For this review, take the finished solid that the model builds, in its own axes (mm). A direction names the side the tool comes from. Give positions to 0.01 mm unless a question says otherwise; leave off trailing zeros. Write each loop counter-clockwise with the first axis right and the second up, starting at its lowest first coordinate (ties: lowest second). Pieces come first, ordered by that corner, then holes. Notation, with made-up numbers: M 39.25,58.5 L 57.25,58.5 A15 ccw 57.25,84.5 Z; hole C 89,60 d4. An arc over 180 degrees is marked long. Answer as a JSON object with one key per item and string values. Group by question number.
```python
from build123d import *

# Parameters (mm, degrees)
SKETCH3_W           = 38.1
SKETCH3_H           = 38.1
BOSS_EXTRUDE2_DEPTH = 3.81
FILLET1_R           = 3.175
CUT_EXTRUDE1_REACH  = 61.178
SKETCH4_R           = 1.627
FILLET2_R           = 1.27
CUT_EXTRUDE2_REACH  = 60.809
SKETCH5_R           = 1.905


with BuildPart() as part:
    # Sketch3 → Boss-Extrude2 (new, symmetric)
    with BuildSketch(Plane.XY):
        Polygon((34.29, -3.175), (34.29, 3.175), (26.67, 3.175), (26.67, 41.275), (34.29, 41.275), (34.29, 47.625), (-34.29, 47.625), (-34.29, 41.275), (-26.67, 41.275), (-26.67, 3.175), (-34.29, 3.175), (-34.29, -3.175), (-19.05, -3.175), (-19.05, 0), (19.05, 0), (19.05, -3.175), align=None)
        with Locations((0, 22.225)):
            Rectangle(SKETCH3_W, SKETCH3_H, mode=Mode.SUBTRACT)
    extrude(amount=BOSS_EXTRUDE2_DEPTH, both=True)

    # Fillet1
    fillet1_edges = [part.edges().sort_by_distance(p)[0] for p in [
        (34.29, 3.175, 0),
        (34.29, 41.275, 0),
        (34.29, 47.625, 0),
        (-34.29, 3.175, 0),
        (-34.29, 41.275, 0),
        (-34.29, 47.625, 0),
        (34.29, -3.175, 0),
        (-34.29, -3.175, 0),
    ]]
    fillet(fillet1_edges, radius=FILLET1_R - 0.0001)  # a hair under: the kernel refuses the full size

    # Sketch4 → Cut-Extrude1 (cut, up to next)
    with BuildSketch(Plane.XY.offset(3.81), mode=Mode.PRIVATE) as cut_extrude1_sk1:
        with Locations((-31.115, 44.45)):
            Circle(SKETCH4_R)
    cut_extrude1_tool1 = extrude(cut_extrude1_sk1.sketch, amount=-CUT_EXTRUDE1_REACH, mode=Mode.PRIVATE) & part.part
    # Sketch4 → Cut-Extrude1 (cut, up to next)
    with BuildSketch(Plane.XY.offset(3.81), mode=Mode.PRIVATE) as cut_extrude1_sk2:
        with Locations((-31.115, 0)):
            Circle(SKETCH4_R)
    cut_extrude1_tool2 = extrude(cut_extrude1_sk2.sketch, amount=-CUT_EXTRUDE1_REACH, mode=Mode.PRIVATE) & part.part
    cut_extrude1_1 = cut_extrude1_tool1.solids().sort_by_distance((-31.115, 44.45, 3.81))[0]
    add(cut_extrude1_1, mode=Mode.SUBTRACT)
    cut_extrude1_2 = cut_extrude1_tool2.solids().sort_by_distance((-31.115, 0, 3.81))[0]
    add(cut_extrude1_2, mode=Mode.SUBTRACT)
    cut_extrude1 = cut_extrude1_1 + cut_extrude1_2  # Cut-Extrude1 as one shape, for the pattern or mirror that repeats it

    # Mirror1: Cut-Extrude1 across plane
    add(cut_extrude1.mirror(Plane(origin=(0, 0, 0), x_dir=(0, 0, 1), z_dir=(1, 0, 0))), mode=Mode.SUBTRACT)

    # Fillet2
    fillet2_edges = [part.edges().sort_by_distance(p)[0] for p in [
        (0, 3.175, 3.81),
        (0, 3.175, -3.81),
        (0, 41.275, 3.81),
        (0, 41.275, -3.81),
        (19.05, 41.275, 0),
        (19.05, 22.225, 3.81),
        (19.05, 3.175, 0),
        (19.05, 22.225, -3.81),
        (-19.05, 3.175, 0),
        (-19.05, 22.225, 3.81),
        (-19.05, 41.275, 0),
        (-19.05, 22.225, -3.81),
        (26.67, 22.225, 3.81),
        (26.67, 22.225, -3.81),
        (-26.67, 22.225, -3.81),
        (-26.67, 22.225, 3.81),
    ]]
    fillet(fillet2_edges, radius=FILLET2_R)

    # Sketch5 → Cut-Extrude2 (cut, up to next)
    with BuildSketch(Plane.XZ, mode=Mode.PRIVATE) as cut_extrude2_sk1:
        with Locations((-15.24, 0)):
            Circle(SKETCH5_R)
    cut_extrude2_tool1 = extrude(cut_extrude2_sk1.sketch, amount=-CUT_EXTRUDE2_REACH, mode=Mode.PRIVATE) & part.part
    # Sketch5 → Cut-Extrude2 (cut, up to next)
    with BuildSketch(Plane.XZ, mode=Mode.PRIVATE) as cut_extrude2_sk2:
        with Locations(Location((15.24, 0, 0), (0, 0, 180))):
            Circle(SKETCH5_R)
    cut_extrude2_tool2 = extrude(cut_extrude2_sk2.sketch, amount=-CUT_EXTRUDE2_REACH, mode=Mode.PRIVATE) & part.part
    add(cut_extrude2_tool1.solids().sort_by_distance((-15.24, 0, 0))[0], mode=Mode.SUBTRACT)
    add(cut_extrude2_tool2.solids().sort_by_distance((15.24, 0, 0))[0], mode=Mode.SUBTRACT)


solid = part.part
```
Item 1: Consider section C-C (x = -0.5). Give the boundary of the cut face in (y, z) (3 decimals).
Item 2: Consider section A-A (x = -15.24). Give the boundary of the cut face in (y, z) (3 decimals).
Item 3: Draft analysis for pull direction X (two halves, no side actions). For faces 1 (the flat face through (-19.05, -2, 0)), 2 (the flat face through (0, 47.625, 0)), 3 (the cylindrical face through (33.385, -2.22, -0.053)), 4 (the cylindrical face through (-33.385, 2.22, -0.053)), state which applies: released by +X, released by -X, zero draft, split by the parting line, or undercut.
Item 4: Machinability: for faces 5 (the cylindrical face through (33.385, 42.23, 0.053)), 6 (the flat face through (0, 41.275, 0)), 7 (the flat face through (19.05, -2, 0)), which of the approach directions +Z, -Z, +X, -X, +Y, -Y give a long, thin tool a straight path to every point of the face, cutting with its end or side? Answer none if there is none.
Item 5: To check wall thickness, follow probe 1 along Z at (x, y) = (15, 2); probe 2 along X at (y, z) = (14.5, 1.5); probe 3 along Y at (x, z) = (31, 3) (3 decimals). State the ranges of each line that lie inside material, in increasing order.
Item 6: Consider section D-D (z = 1). State how many separate pieces and enclosed holes the cut face has, plus the area to 3 significant figures.
Item 7: Consider section B-B (y = 36.5). Give the boundary of the cut face in (x, z), plus the area to 3 significant figures.
Item 8: Insertion check: P1, Ø4, axis at x = -31.115, y = 44.45, coming from the -Z side; P2, Ø4, axis at y = 27, z = -1, coming from the +X side; P3, Ø4, axis at x = 9, z = 0, coming from the -Y side; P4, Ø1, axis at y = -2, z = 0.5, coming from the -X side. Each pin has a flat end and moves straight along its axis. Give the tip position at first contact, or say it passes through.
Result set:
{
 "1": {"outline": "M 0,-3.81 L 1.905,-3.81 A1.27 ccw 3.175,-2.54 L 3.175,2.54 A1.27 ccw 1.905,3.81 L 0,3.81 Z; M 41.275,-2.54 A1.27 ccw 42.545,-3.81 L 47.625,-3.81 L 47.625,3.81 L 42.545,3.81 A1.27 ccw 41.275,2.54 Z"},
 "2": {"outline": "M 0,-3.81 L 1.905,-3.81 A1.27 ccw 3.175,-2.54 L 3.175,-1.905 L 0,-1.905 Z; M 0,1.905 L 3.175,1.905 L 3.175,2.54 A1.27 ccw 1.905,3.81 L 0,3.81 Z; M 41.275,-2.54 A1.27 ccw 42.545,-3.81 L 47.625,-3.81 L 47.625,3.81 L 42.545,3.81 A1.27 ccw 41.275,2.54 Z"},
 "3": {"face 1": "undercut", "face 2": "zero draft", "face 3": "released by +X", "face 4": "released by -X"},
 "4": {"face 5": "+Z, -Z, +X", "face 6": "+Z, -Z", "face 7": "+Z, -Z, -Y"},
 "5": {"probe 1": "z = -3.81 to -1.89, 1.89 to 3.81", "probe 2": "x = -26.67 to -19.05, 19.05 to 26.67", "probe 3": "y = -3.175 to -1.623, 1.623 to 3.175, 41.275 to 42.827, 46.073 to 47.625"},
 "6": {"separate pieces": "2", "enclosed holes": "4", "area": "1,260 mm^2"},
 "7": {"outline": "M -26.67,-2.54 A1.27 ccw -25.4,-3.81 L -20.32,-3.81 A1.27 ccw -19.05,-2.54 L -19.05,2.54 A1.27 ccw -20.32,3.81 L -25.4,3.81 A1.27 ccw -26.67,2.54 Z; M 19.05,-2.54 A1.27 ccw 20.32,-3.81 L 25.4,-3.81 A1.27 ccw 26.67,-2.54 L 26.67,2.54 A1.27 ccw 25.4,3.81 L 20.32,3.81 A1.27 ccw 19.05,2.54 Z", "area": "113 mm^2"},
 "8": {"P1": "stops at z = -3.81", "P2": "stops at x = 26.67", "P3": "stops at y = 0", "P4": "stops at x = -33.91"}
}
